Can you work these out from the model? Positions are in its coordinate system, mm. A direction names the side the tool comes from. Coordinates: 2 decimals unless noted, no trailing zeros. Write each loop counter-clockwise with the first axis right and the second up, starting at its lowest first coordinate (ties: lowest second). Pieces come first, ordered by that corner, then holes. Notation, with made-up numbers: (-27.5, -11) -> (17.5, -11) arc R29 cw to (17.5, 25) -> close; hole circle Ø6 at (60.25, 42.5). An arc over 180 degrees is marked (long way). Use one line per item in the form item = value.
Autodesk Inventor part; units mm, degrees
ref_plane "YZ Plane" through (0, 0, 0) normal (1, 0, 0) x (0, 1, 0)
ref_plane "XZ Plane" through (0, 0, 0) normal (0, 1, 0) x (-1, 0, 0)
ref_plane "XY Plane" through (0, 0, 0) normal (0, 0, 1) x (1, 0, 0)
sketch "Sketch1" plane through (0, 0, 0) normal (0, 0, 1) x (1, 0, 0)
  line L0 (-10, -27.5) -> (10, -27.5)
  line L1 (10, -27.5) -> (10, 27.5)
  line L2 (10, 27.5) -> (-10, 27.5)
  line L3 (-10, 27.5) -> (-10, -27.5)
  line L4 (-10, -27.5) -> (10, 27.5) construction
  line L5 (10, -27.5) -> (-10, 27.5) construction
  point P0 (0, 0)
  dimension "d0" = 20
  dimension "d1" = 55
extrude "Extrusion1" add sketch "Sketch1" along normal blind 10
sketch "Sketch3" plane through (10, -27.5, 0) normal (1, 0, 0) x (0, 0, -1)
  line L0 (0, 0) -> (0, 55) construction
  line L1 (-10, 0) -> (-10, 55)
  line L2 (-10, 55) -> (-20, 65)
  line L3 (0, 55) -> (-10, 55)
  line L4 (-20, 65) -> (0, 65)
  line L5 (0, 65) -> (0, 55)
  line L6 (0, 27.5) -> (-50, 27.5) construction
  line L7 (-10, 0) -> (-20, -10)
  line L8 (0, 0) -> (-10, 0)
  line L9 (-20, -10) -> (0, -10)
  line L10 (0, -10) -> (0, 0)
  dimension "d8" = 20
  dimension "d12" = 10
  dimension "d13" = 50
extrude "Extrusion3" add sketch "Sketch3" against normal blind 20
sketch "Sketch4" plane through (0, 0, 10) normal (0, 0, 1) x (1, 0, 0)
  circle A0 centre (0, 20) radius 2.5
  circle A1 centre (0, 0) radius 2.5
  circle A2 centre (0, -20) radius 2.5
  dimension "d14" = 5
  dimension "d15" = 5
  dimension "d16" = 5
  dimension "d17" = 20
  dimension "d18" = 20
sketch "Sketch5" plane through (10, -37.5, 0) normal (0, -1, 0) x (1, 0, 0)
  circle A0 centre (-10, 7.5) radius 2.5
  circle A1 centre (-10, 7.5) radius 2.5
  point P0 (-10, 0)
  dimension "d19" = 5
  dimension "d20" = 7.5
  dimension "d35" = 5
extrude "Extrusion4" cut sketch "Sketch5" against normal blind 10
extrude "Extrusion5" cut sketch "Sketch4" against normal through all
thread "Thread1"
thread "Thread2"
thread "Thread3"
thread "Thread4"
thread "Thread5"
sketch "Sketch6" plane through (10, 37.5, 20) normal (0, 1, 0) x (1, 0, 0)
  circle A0 centre (-10, 12.5) radius 2.5
  line L0 (0, 20) -> (0, 0)
  point P0 (-10, 20)
  dimension "d36" = 5
  dimension "d37" = 7.5
  dimension "d38" = 10
extrude "Extrusion6" cut sketch "Sketch6" against normal blind 10
thread "Thread6"
sketch "Sketch7" plane through (10, 37.5, 20) normal (1, 0, 0) x (0, 0, -1)
  circle A0 centre (15, -27.5) radius 2.5
  circle A1 centre (15, -47.5) radius 2.5
  line L0 (20, -35) -> (20, -40)
  line L1 (10, -40) -> (10, -35)
  line L2 (20, -75) -> (20, 0)
  point P0 (20, -37.5)
  dimension "d43" = 5
  dimension "d44" = 5
  dimension "d45" = 20
  dimension "d46" = 7.5
  dimension "d47" = 5
  dimension "d48" = 5
extrude "Extrusion7" cut sketch "Sketch7" against normal through all
thread "Thread7"
thread "Thread8"
sketch "Sketch8" plane through (10, 37.5, 20) normal (0, 1, 0) x (1, 0, 0)
  circle A0 centre (-225, 20) radius 225
  line L0 (0, 20) -> (-20, 20)
  circle A1 centre (-225, 20) radius 230
  point P0 (-10, 20)
  point P1 (-10, 20)
  dimension "d55" = 450
  dimension "d56" = 5
extrude "Extrusion8" cut sketch "Sketch8" against normal through all
sketch "Sketch9" plane through (-10, 37.5, 20) normal (0, 1, 0) x (1, 0, 0)
  circle A0 centre (225, 20) radius 225
  circle A1 centre (225, 20) radius 230
  point P0 (10, 20)
  point P1 (0, 20)
  dimension "d59" = 450
  dimension "d60" = 5
extrude "Extrusion9" cut sketch "Sketch9" against normal through all
properties material "ABS Plastic"
Q1. Will these pins go through, and if not, where does the flat tip stop? pin 1 (6.5 mm diameter, centred on x = 0, y = -20, fed in from +Z); pin 2 (3 mm diameter, centred on x = 0, z = 7.5, fed in from -Y); pin 3 (6 mm diameter, centred on y = -10, z = 5, fed in from -X).
Return value:
pin_1 = 10
pin_2 = -27.5
pin_3 = -9.99
Q2. Suppose I cut it at A-A (y = 20). Write out the boundary of the cut face in (x, z).
Return value:
outline = (-10, 0) -> (-2.5, 0) -> (-2.5, 10) -> (-9.78, 10) arc R225 ccw to start; (2.5, 0) -> (10, 0) arc R225 ccw to (9.78, 10) -> (2.5, 10) -> close
Q3. Suppose I cut it at C-C (x = -3.25). Write out the boundary of the cut face in (y, z), then the cut area to 3 significant figures.
Return value:
outline = (-37.5, 0) -> (37.5, 0) -> (37.5, 20) -> (27.5, 10) -> (-27.5, 10) -> (-37.5, 20) -> close; hole circle Ø5 at (-10, 5); hole circle Ø5 at (10, 5)
area = 811 mm2
Q4. Thinking about a two-plate mould opening in Z: for faces 4 (the cylindrical face through (1.34, -17.89, 5.07)), 5 (the flat face through (0, 27.5, 7)), 6 (the flat face through (4, 1, 0)), 7 (the flat face through (0.1, -32.4, 14.9)), which applies, released by +Z, released by -Z, zero draft, split by the parting line, or undercut?
Return value:
face_4 = zero draft
face_5 = undercut
face_6 = released by -Z
face_7 = released by +Z
Q5. Suppose I cut it at B-B (z = 3.5). Write out the boundary of the cut face in (x, y).
Return value:
outline = (-9.97, -37.5) -> (9.97, -37.5) -> (9.97, -12) -> (-9.97, -12) -> close; (-9.97, -8) -> (9.97, -8) -> (9.97, 8) -> (-9.97, 8) -> close; (-9.97, 12) -> (9.97, 12) -> (9.97, 37.5) -> (-9.97, 37.5) -> close; hole circle Ø5 at (0, -20); hole circle Ø5 at (0, 0); hole circle Ø5 at (0, 20)
Q6. For faces 1 (the cylindrical face through (-0.54, 32.57, 9.94)), 2 (the flat face through (0, -27.5, 8)), 3 (the flat face through (0.1, 32.4, 14.9)), which set-ups out of +Z, -Z, +X, -X, +Y, -Y let a thin tool reach every point of the face, with its end or its side?
Return value:
face_1 = +Y
face_2 = -Y
face_3 = +Z, +X, -X
Q7. If I drill on line 1 (Y direction, x = -4, z = 5); line 2 (Y direction, x = 9, z = 7.25); line 3 (Z direction, x = 4.75, y = -10), over which ranges is the centre line in solid material (lowest first)? Write a range as from..to.
Return value:
line_1 = -37.5..-12.5, -7.5..7.5, 12.5..37.5
line_2 = -37.5..-11.09, -8.91..8.91, 11.09..37.5
line_3 = 0..2.5, 7.5..10
Q8. Suppose I cut it at D-D (z = 14). Write out the boundary of the cut face in (x, y), then the cut area to 3 significant figures.
Return value:
outline = (-9.56, -37.5) -> (9.56, -37.5) -> (9.56, -31.5) -> (-9.56, -31.5) -> close; (-9.56, 31.5) -> (9.56, 31.5) -> (9.56, 37.5) -> (-9.56, 37.5) -> close
area = 230 mm2
